from build123d import *

# Parameters (mm, degrees)
SKETCH_1_R          = 3.75
EXTRUDE_1_DEPTH     = 1
SKETCH_2_R          = 3
EXTRUDE_2_DEPTH     = 10
SKETCH_3_R          = 2.1
CUT_EXTRUDE_1_DEPTH = 13.211674742
CHAMFER_1_SIZE      = 0.2
CHAMFER_2_SIZE      = 0.2


with BuildPart() as part:
    # 草图1 → 凸台-拉伸1 (new body)
    with BuildSketch(Plane(origin=(0, 0, 0), x_dir=(1, 0, 0), z_dir=(0, 1, 0))):
        with Locations(Location((0, 0, 0), (0, 0, 270))):
            Circle(SKETCH_1_R)
    extrude(amount=EXTRUDE_1_DEPTH)

    # 草图2 → 凸台-拉伸2 (add)
    with BuildSketch(Plane(origin=(0, 1, 0), x_dir=(1, 0, 0), z_dir=(0, 1, 0))):
        with Locations(Location((0, 0, 0), (0, 0, 270))):
            Circle(SKETCH_2_R)
    extrude(amount=EXTRUDE_2_DEPTH)

    # 草图3 → 切除-拉伸1 (cut, through all)
    with BuildSketch(Plane(origin=(0, 11, 0), x_dir=(1, 0, 0), z_dir=(0, 1, 0))):
        with Locations(Location((0, 0, 0), (0, 0, 270))):
            Circle(SKETCH_3_R)
    extrude(amount=-CUT_EXTRUDE_1_DEPTH, mode=Mode.SUBTRACT)

    # 倒角1
    chamfer_1_edges = [part.edges().sort_by_distance(p)[0] for p in [
        (0, 1, -3.75),
        (0, 11, -3),
    ]]
    chamfer(chamfer_1_edges, length=CHAMFER_1_SIZE)

    # 倒角2
    chamfer_2_edges = [part.edges().sort_by_distance(p)[0] for p in [
        (0, 0, -2.1),
        (0, 11, -2.1),
        (0, 0, -3.75),
    ]]
    chamfer(chamfer_2_edges, length=CHAMFER_2_SIZE)


solid = part.part
Could you check a few things on this model? Use its own coordinates, in mm. Give positions to 0.01 mm unless a question says otherwise; leave off trailing zeros. Order: outer loops, then holes, each group sorted by start corner. A loop starts at its lowest first (then second) coordinate and runs counter-clockwise, first axis right, second up.
1. We'd pull the mould along Z, two halves only. Please class faces 1 (the cylindrical face through (0.9, 5.83, 2.86)), 2 (the cylindrical face through (0.631, 5.574, 2.003)), 3 (the flat face through (3, 1, -1)): pulls with the +Z half, pulls with the -Z half, needs draft (parallel to the pull), parting line crosses it, or undercut.
2. Suppose I cut it at C-C (y = 6.5). List the corners of the cut face in (x, z) for me.
3. Suppose I cut it at B-B (x = 0). List the corners of the cut face in (y, z) for me, plus the area to 3 significant figures.
4. I need wall thicknesses on L1, parallel to X at y = 7.5, z = 0; L2, parallel to Z at x = 0.25, y = 2.25; L3, parallel to Z at x = 1.25, y = 4.5. Which ranges of each line are inside material? Lowest first, please.
5. Will these pins go through, and if not, where does the flat tip stop? P1, Ø4, axis at y = 5.5, z = 0, coming from the +X side; P2, Ø4, axis at x = -2, y = 6.5, coming from the +Z side; P3, Ø3.5, axis at x = 0, z = 0, coming from the -Y side.
6. Suppose I cut it at A-A (z = 0). List the corners of the cut face in (x, y) for me, plus the area to 3 significant figures.
Solved:
1. face 1: parting line crosses it
1. face 2: undercut
1. face 3: needs draft
2. outline: circle Ø6 at (0, 0); hole circle Ø4.2 at (0, 0)
3. outline: (0, -3.55) - (0.2, -3.75) - (0.8, -3.75) - (1, -3.55) - (1, -3) - (10.8, -3) - (11, -2.8) - (11, -2.3) - (10.8, -2.1) - (0.2, -2.1) - (0, -2.3) - close; (0, 2.3) - (0.2, 2.1) - (10.8, 2.1) - (11, 2.3) - (11, 2.8) - (10.8, 3) - (1, 3) - (1, 3.55) - (0.8, 3.75) - (0.2, 3.75) - (0, 3.55) - close
3. area: 21.1 mm2
4. L1: x = -3 to -2.1, 2.1 to 3
4. L2: z = -2.99 to -2.09, 2.09 to 2.99
4. L3: z = -2.73 to -1.69, 1.69 to 2.73
5. P1: stops at x = 3
5. P2: stops at z = 3
5. P3: passes through
6. outline: (-3.75, 0.2) - (-3.55, 0) - (-2.3, 0) - (-2.1, 0.2) - (-2.1, 10.8) - (-2.3, 11) - (-2.8, 11) - (-3, 10.8) - (-3, 1) - (-3.55, 1) - (-3.75, 0.8) - close; (2.1, 0.2) - (2.3, 0) - (3.55, 0) - (3.75, 0.2) - (3.75, 0.8) - (3.55, 1) - (3, 1) - (3, 10.8) - (2.8, 11) - (2.3, 11) - (2.1, 10.8) - close
6. area: 21.1 mm2
